from build123d import *

# Parameters (mm, degrees)
SKETCH1_W           = 80
SKETCH1_H           = 50
BOSS_EXTRUDE1_DEPTH = 85
SKETCH3_W           = 50
SKETCH3_H           = 55.289699502
CUT_EXTRUDE1_DEPTH  = 40
SKETCH4_R           = 7.5
CUT_EXTRUDE3_DEPTH  = 120.373363863
CUT_EXTRUDE4_DEPTH  = 107.418983269


with BuildPart() as part:
    # Sketch1 → Boss-Extrude1 (new body)
    with BuildSketch(Plane.XY):
        Rectangle(SKETCH1_W, SKETCH1_H)
    extrude(amount=BOSS_EXTRUDE1_DEPTH)

    # Sketch3 → Cut-Extrude1 (cut)
    with BuildSketch(Plane(origin=(0, 0, 0), x_dir=(-1, 0, 0), z_dir=(0, 0, -1))):
        Rectangle(SKETCH3_W, SKETCH3_H)
    extrude(amount=-CUT_EXTRUDE1_DEPTH, mode=Mode.SUBTRACT)

    # Sketch4 → Cut-Extrude3 (cut, through all)
    with BuildSketch(Plane(origin=(40, 0, 0), x_dir=(0, 0, -1), z_dir=(1, 0, 0))):
        with Locations((-15, 0)):
            Circle(SKETCH4_R)
    extrude(amount=-CUT_EXTRUDE3_DEPTH, mode=Mode.SUBTRACT)

    # Sketch5 → Cut-Extrude4 (cut, through all)
    with BuildSketch(Plane(origin=(0, 25, 0), x_dir=(1, 0, 0), z_dir=(0, 1, 0))):
        with BuildLine():
            Line((25, -40), (-25, -40))
            ThreePointArc((-25, -40), (0, -65), (25, -40))
        make_face()
    extrude(amount=-CUT_EXTRUDE4_DEPTH, mode=Mode.SUBTRACT)


solid = part.part
Source: CAD feature listing. Evaluate the final solid. Frame: model axes, mm. A direction names the side the tool comes from. Give positions to 0.01 mm unless a question says otherwise; leave off trailing zeros. Order: outer loops, then holes, each group sorted by start corner. A loop starts at its lowest first (then second) coordinate and runs counter-clockwise, first axis right, second up. Notation, with made-up numbers: (0, -12) -> (29, -12) arc R18 cw to (29, 2) -> close; hole circle Ø6 at (-21.5, -32.75). An arc over 180 degrees is marked (long way). Write item = value, one per line.
Item 1: Section query D-D (x = -10). Output: boundary loops of the cut face in (y, z).
Check result:
outline = (-25, 62.91) -> (25, 62.91) -> (25, 85) -> (-25, 85) -> close
Item 2: Mould query, pull axis Y, two halves, no side actions, for faces 3 (the face through (-32.395, 0.33, 22.493)), 4 (the face through (-1, -25, 70)), 5 (the face through (-1, 0, 85)). Classes: +Y half, -Y half, draft (parallel to the pull), parting line (faces both ways), or undercut.
Check result:
face_3 = undercut
face_4 = -Y half
face_5 = draft
Item 3: Section query A-A (z = 27). Output: boundary loops of the cut face in (x, y), then the cut area to 3 significant figures.
Check result:
outline = (-40, -25) -> (-25, -25) -> (-25, 25) -> (-40, 25) -> close; (25, -25) -> (40, -25) -> (40, 25) -> (25, 25) -> close
area = 1,500 mm²
Item 4: Section query C-C (z = 15). Output: boundary loops of the cut face in (x, y), then the cut area to 3 significant figures.
Check result:
outline = (-40, -25) -> (-25, -25) -> (-25, -7.5) -> (-40, -7.5) -> close; (-40, 7.5) -> (-25, 7.5) -> (-25, 25) -> (-40, 25) -> close; (25, -25) -> (40, -25) -> (40, -7.5) -> (25, -7.5) -> close; (25, 7.5) -> (40, 7.5) -> (40, 25) -> (25, 25) -> close
area = 1,050 mm²
Item 5: Section query B-B (y = 0). Output: boundary loops of the cut face in (x, z).
Check result:
outline = (-40, 0) -> (-25, 0) -> (-25, 7.5) -> (-40, 7.5) -> close; (-40, 22.5) -> (-25, 22.5) -> (-25, 40) arc R25 cw to (25, 40) -> (25, 22.5) -> (40, 22.5) -> (40, 85) -> (-40, 85) -> close; (25, 0) -> (40, 0) -> (40, 7.5) -> (25, 7.5) -> close
Item 6: Ray query, probe 1 along X at (y, z) = (3, 27.5); probe 2 along Y at (x, z) = (35.5, 15); probe 3 along X at (y, z) = (3, 57.5). Return the intervals inside material, ascending.
Check result:
probe_1 = -40 to -25, 25 to 40
probe_2 = -25 to -7.5, 7.5 to 25
probe_3 = -40 to -17.85, 17.85 to 40
Item 7: Set-up query: faces 1 (the face through (40, 0, 42)), 2 (the face through (25, 0, 24)). Return all of +Z, -Z, +X, -X, +Y, -Y with unobstructed straight access to the full face (end or side cutting, diameter ignored); none if empty.
Check result:
face_1 = +Z, -Z, +X, +Y, -Y
face_2 = -Z, +Y, -Y
Item 8: Contact query for flat-ended pins moving along their axis: pin 1 (19.5 mm diameter, centred on y = 0, z = 15, fed in from +X); pin 2 (6 mm diameter, centred on x = -16, y = -17.5, fed in from -Z). Output: stop coordinate, or through.
Check result:
pin_1 = 40
pin_2 = 56.25
